Answer from the drawing. Dimensions are ordinates in mm from the lowest x, y and z of the part. A direction names the side the tool comes from. Coordinates: 2 decimals unless noted, no trailing zeros. Order: outer loops, then holes, each group sorted by start corner. A loop starts at its lowest first (then second) coordinate and runs counter-clockwise, first axis right, second up. Notation, with made-up numbers: M -7,83.25 L 0,83.25 A31 cw 0,121.25 Z; hole C 51.25,7.25 d1. An arc over 180 degrees is marked long. Write each question's results on one line, items separated by ' | '.
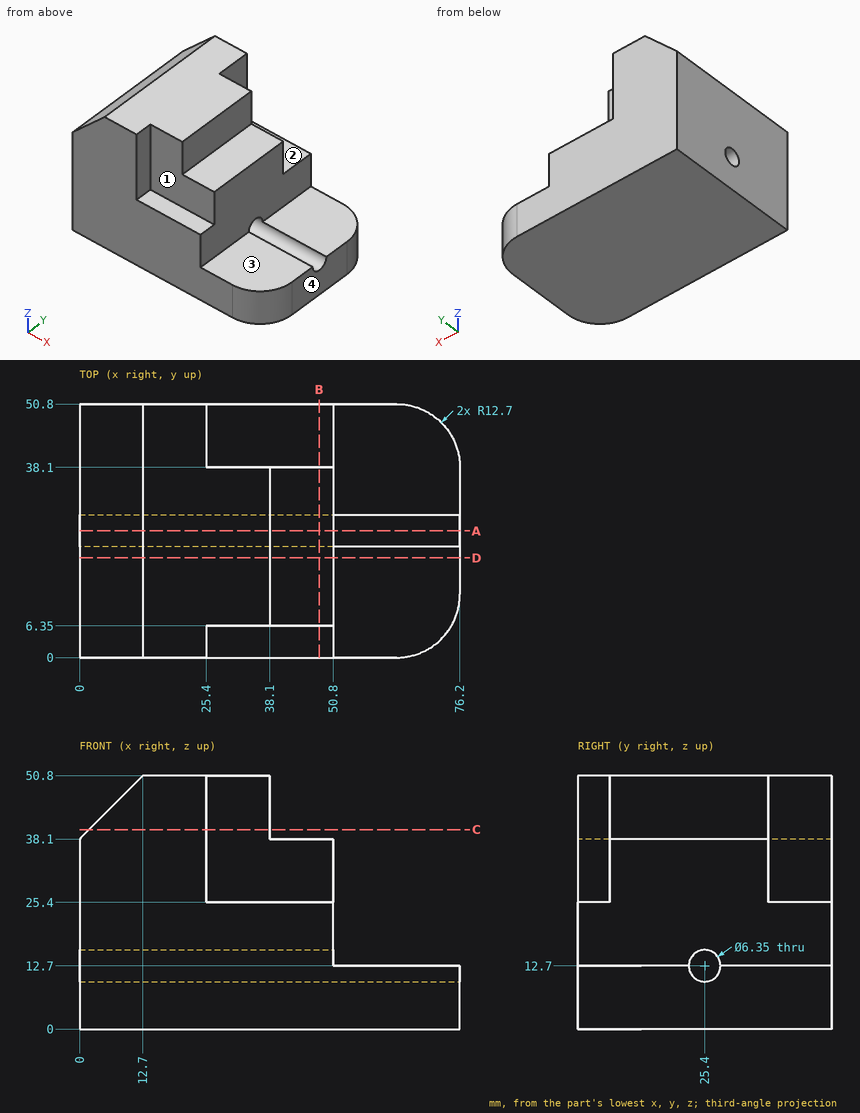
(1) The part is cut by section C-C, the plane z = 40. Write down the section's boundary in (x, y), then the cut area to 3 significant figures.
Conclusion:
outline: M 1.9,0 L 25.4,0 L 25.4,6.35 L 38.1,6.35 L 38.1,38.1 L 25.4,38.1 L 25.4,50.8 L 1.9,50.8 Z | area: 1,600 mm²
(2) Straight lines are drawn through the part: line 1 (Y direction, x = 28, z = 12.7) (3 decimals); line 2 (Z direction, x = 26, y = 25.4) (3 decimals); line 3 (Z direction, x = 49, y = 25.4) (3 decimals). For each, find the intervals that lie inside material, in ascending order.
Conclusion:
line 1: 0 to 22.225, 28.575 to 50.8 | line 2: 0 to 9.525, 15.875 to 50.8 | line 3: 0 to 9.525, 15.875 to 38.1
(3) Given pin 1 (1.9 mm diameter, centred on y = 4, z = 37, fed in from +X); pin 2 (10 mm diameter, centred on x = 64.5, y = 31.5, fed in from +Z); pin 3 (4 mm diameter, centred on y = 23.5, z = 43, fed in from +X); pin 4 (5 mm diameter, centred on y = 25.4, z = 12.7, fed in from -X), each flat-ended and moving along its own axis, determine where each tip first touches the part or whether it passes through.
Conclusion:
pin 1: x = 25.4 | pin 2: z = 12.7 | pin 3: x = 38.1 | pin 4: through
(4) The part is cut by section D-D, the plane y = 20. Write down the section's boundary in (x, z), then the cut area to 3 significant figures.
Conclusion:
outline: M 0,0 L 76.2,0 L 76.2,12.7 L 50.8,12.7 L 50.8,38.1 L 38.1,38.1 L 38.1,50.8 L 12.7,50.8 L 0,38.1 Z | area: 2,660 mm²
(5) For the marked faces 1, 2, 3 and 4, determine the directions among +Z, -Z, +X, -X, +Y, -Y from which every point of the face is accessible in a straight line to the end or side of a thin tool.
Conclusion:
face 1: +Z, +X, -Y | face 2: +Z, +X, +Y | face 3: +Z, +X, +Y, -Y | face 4: +Z, -Z, +X, +Y, -Y
(6) The part is cut by section A-A, the plane y = 25.4. Write down the section's boundary in (x, z) (3 decimals), then the cut area to 3 significant figures.
Conclusion:
outline: M 0,0 L 76.2,0 L 76.2,9.525 L 0,9.525 Z; M 0,15.875 L 50.8,15.875 L 50.8,38.1 L 38.1,38.1 L 38.1,50.8 L 12.7,50.8 L 0,38.1 Z | area: 2,260 mm²
(7) The part is cut by section B-B, the plane x = 48. Write down the section's boundary in (y, z) (3 decimals).
Conclusion:
outline: M 0,0 L 50.8,0 L 50.8,25.4 L 38.1,25.4 L 38.1,38.1 L 6.35,38.1 L 6.35,25.4 L 0,25.4 Z; hole C 25.4,12.7 d6.35
